Autodesk Inventor part; units mm, degrees
ref_plane "YZ Plane" through (0, 0, 0) normal (1, 0, 0) x (0, 1, 0)
ref_plane "XZ Plane" through (0, 0, 0) normal (0, 1, 0) x (-1, 0, 0)
ref_plane "XY Plane" through (0, 0, 0) normal (0, 0, 1) x (1, 0, 0)
sketch "Sketch_1" plane through (0, 0, 0) normal (0, 0, 1) x (1, 0, 0)
  arc A0 (-7.5, 2) -> (-7.2, 1.7) centre (-7.2, 2) ccw
  line L0 (-7.2, 1.7) -> (-6.4, 1.7)
  line L1 (-6.4, 1.7) -> (-6.4, 2.85)
  line L2 (-6.4, 2.85) -> (-3.8, 2.85)
  line L3 (-3.8, 2.85) -> (-2.8, 1.85)
  line L4 (-2.8, 1.85) -> (-2.8, 0.5196)
  line L5 (-2.8, 0.5196) -> (-2.5, 0)
  line L6 (-2.5, 0) -> (-2.8, -0.5196)
  line L7 (-2.8, -0.5196) -> (-2.8, -1.85)
  line L8 (-2.8, -1.85) -> (-3.8, -2.85)
  line L9 (-3.8, -2.85) -> (-6.4, -2.85)
  line L10 (-6.4, -2.85) -> (-6.4, -1.7)
  line L11 (-6.4, -1.7) -> (-7.2, -1.7)
  arc A1 (-7.2, -1.7) -> (-7.5, -2) centre (-7.2, -2) ccw
  line L12 (-7.5, -2) -> (-7.5, -6.5)
  arc A2 (-7.5, -6.5) -> (-6.5, -7.5) centre (-6.5, -6.5) ccw
  line L13 (-6.5, -7.5) -> (-2, -7.5)
  arc A3 (-2, -7.5) -> (-1.7, -7.2) centre (-2, -7.2) ccw
  line L14 (-1.7, -7.2) -> (-1.7, -6.4)
  line L15 (-1.7, -6.4) -> (-2.85, -6.4)
  line L16 (-2.85, -6.4) -> (-2.85, -3.8)
  line L17 (-2.85, -3.8) -> (-1.85, -2.8)
  line L18 (-1.85, -2.8) -> (-0.5196, -2.8)
  line L19 (-0.5196, -2.8) -> (0, -2.5)
  line L20 (0, -2.5) -> (0.5196, -2.8)
  line L21 (0.5196, -2.8) -> (1.85, -2.8)
  line L22 (1.85, -2.8) -> (2.85, -3.8)
  line L23 (2.85, -3.8) -> (2.85, -6.4)
  line L24 (2.85, -6.4) -> (1.7, -6.4)
  line L25 (1.7, -6.4) -> (1.7, -7.2)
  arc A4 (1.7, -7.2) -> (2, -7.5) centre (2, -7.2) ccw
  line L26 (2, -7.5) -> (6.5, -7.5)
  arc A5 (6.5, -7.5) -> (7.5, -6.5) centre (6.5, -6.5) ccw
  line L27 (7.5, -6.5) -> (7.5, -2)
  arc A6 (7.5, -2) -> (7.2, -1.7) centre (7.2, -2) ccw
  line L28 (7.2, -1.7) -> (6.4, -1.7)
  line L29 (6.4, -1.7) -> (6.4, -2.85)
  line L30 (6.4, -2.85) -> (3.8, -2.85)
  line L31 (3.8, -2.85) -> (2.8, -1.85)
  line L32 (2.8, -1.85) -> (2.8, -0.5196)
  line L33 (2.8, -0.5196) -> (2.5, 0)
  line L34 (2.5, 0) -> (2.8, 0.5196)
  line L35 (2.8, 0.5196) -> (2.8, 1.85)
  line L36 (2.8, 1.85) -> (3.8, 2.85)
  line L37 (3.8, 2.85) -> (6.4, 2.85)
  line L38 (6.4, 2.85) -> (6.4, 1.7)
  line L39 (6.4, 1.7) -> (7.2, 1.7)
  arc A7 (7.2, 1.7) -> (7.5, 2) centre (7.2, 2) ccw
  line L40 (7.5, 2) -> (7.5, 6.5)
  arc A8 (7.5, 6.5) -> (6.5, 7.5) centre (6.5, 6.5) ccw
  line L41 (6.5, 7.5) -> (2, 7.5)
  arc A9 (2, 7.5) -> (1.7, 7.2) centre (2, 7.2) ccw
  line L42 (1.7, 7.2) -> (1.7, 6.4)
  line L43 (1.7, 6.4) -> (2.85, 6.4)
  line L44 (2.85, 6.4) -> (2.85, 3.8)
  line L45 (2.85, 3.8) -> (1.85, 2.8)
  line L46 (1.85, 2.8) -> (0.5196, 2.8)
  line L47 (0.5196, 2.8) -> (0, 2.5)
  line L48 (0, 2.5) -> (-0.5196, 2.8)
  line L49 (-0.5196, 2.8) -> (-1.85, 2.8)
  line L50 (-1.85, 2.8) -> (-2.85, 3.8)
  line L51 (-2.85, 3.8) -> (-2.85, 6.4)
  line L52 (-2.85, 6.4) -> (-1.7, 6.4)
  line L53 (-1.7, 6.4) -> (-1.7, 7.2)
  arc A10 (-1.7, 7.2) -> (-2, 7.5) centre (-2, 7.2) ccw
  line L54 (-2, 7.5) -> (-6.5, 7.5)
  arc A11 (-6.5, 7.5) -> (-7.5, 6.5) centre (-6.5, 6.5) ccw
  line L55 (-7.5, 6.5) -> (-7.5, 2)
  circle A12 centre (0, 0) radius 1.25
extrude "Extrusion1" add sketch "Sketch_1" along normal blind 150
equation "\"d0\" = L"
equation "\"L\" = 150"
properties part number "HFS3-1515-150" material "アルミニウム 6061"
Input: part model. Units: mm. Frame: model coordinates. A direction names the side the tool comes from. Give positions to 0.01 mm unless a question says otherwise; leave off trailing zeros.
1. Set-up query: faces 4 (the face through (-5, -2.85, 74)), 5 (the face through (7.5, 4, 74)). Return all of +Z, -Z, +X, -X, +Y, -Y with unobstructed straight access to the full face (end or side cutting, diameter ignored); none if empty.
Computed:
face 4: +Z, -Z
face 5: +Z, -Z, +X, +Y, -Y
2. Pin query (flat end, axial travel): pin 1 Ø0.9 at (y, z) = (7, 106) entering from +X; pin 2 Ø0.6 at (x, z) = (-7, 106) entering from +Y; pin 3 Ø1.5 at (y, z) = (0.5, 111) entering from +X. Return the tip coordinate at first contact, or that it passes through.
Computed:
pin 1: stops at x = 7.5
pin 2: stops at y = 7.48
pin 3: stops at x = 2.8
3. Line query: probe 1 along Y at (x, z) = (0, 39); probe 2 along Y at (x, z) = (-5, 59.5); probe 3 along X at (y, z) = (-6.5, 129.5). Output: solid intervals per line, ascending.
Computed:
probe 1: y = -2.5 to -1.25, 1.25 to 2.5
probe 2: y = -7.5 to -2.85, 2.85 to 7.5
probe 3: x = -7.5 to -1.7, 1.7 to 7.5
4. Draft query along X for faces 1 (the face through (-4, -7.5, 74)), 2 (the face through (-5, 2.85, 74)), 3 (the face through (7.5, -4, 74)). Return one class per face: released by +X, released by -X, zero draft, split by the parting line, or undercut.
Computed:
face 1: zero draft
face 2: undercut
face 3: released by +X
